```python
from build123d import *

# Parameters (mm, degrees)
F2_R        = 2.8448
F3_DEPTH    = 7.5184
F2_R_2      = 6.35
F4_DEPTH    = 7.5184
F5_R        = 5.08
F6_T1_DEPTH = 7.5184
F9_DEPTH    = 0.508


# Not quite as in the source:
# - a fillet or chamfer that OpenCascade refuses, or shapes differently, is made with other operations: its cross-section is extruded or revolved along the edge and cut away or added
# - two fillets or chamfers of one size are made in one step


with BuildPart() as f1:
    # F0 (on Front) → F1 (revolve)
    with BuildSketch(Plane.XZ):
        with BuildLine():
            Line((32.385, 31.75), (0, 31.75))
            Line((0, 31.75), (0, 28.575))
            Line((0, 28.575), (32.4854701757, 28.575))
            Line((32.4854701757, 28.575), (35.56, 25.49819462))
            Line((35.56, 25.49819462), (35.56, 8.8277412578))
            Line((35.56, 8.8277412578), (39.5224, 4.572))
            Line((39.5224, 4.572), (39.5224, 0))
            Line((39.5224, 0), (43.053, 0))
            Line((43.053, 0), (43.053, -0.508))
            Line((43.053, -0.508), (44.069, -0.508))
            Line((44.069, -0.508), (44.069, 7.5184))
            Line((44.069, 7.5184), (40.8266418362, 7.5184))
            Line((40.8266418362, 7.5184), (38.735, 9.7710676491))
            Line((38.735, 9.7710676491), (38.735, 25.4))
            ThreePointArc((38.735, 25.4), (36.8751280605, 29.8901280605), (32.385, 31.75))
        make_face()
    revolve(axis=Axis((0, 0, 30.1625), (0, 0, 1)))

    # F2 (on face) → F3 (join)
    with BuildSketch(Plane(origin=(0, 0, 0), x_dir=(1, 0, 0), z_dir=(0, 0, -1))):
        with BuildLine():
            ThreePointArc((4.7616218936, 42.7888743243), (5.939646413, 44.7443151405), (6.35, 46.99))
            ThreePointArc((6.35, 46.99), (-2.2456848595, 52.929646413), (-4.7616218936, 42.7888743243))
            ThreePointArc((-4.7616218936, 42.7888743243), (0, 43.053), (4.7616218936, 42.7888743243))
        make_face()
        with Locations((0, 46.99)):
            Circle(F2_R, mode=Mode.SUBTRACT)
    extrude(amount=-F3_DEPTH)

    # F2 (on face) → F4 (join)
    with BuildSketch(Plane(origin=(0, 0, 0), x_dir=(1, 0, 0), z_dir=(0, 0, -1))):
        with Locations((0, 46.99)):
            Circle(F2_R_2)
        with Locations((0, 46.99)):
            Circle(F2_R, mode=Mode.SUBTRACT)
        with Locations((4.699, -46.7544596696)):
            Circle(F2_R_2)
        with Locations((4.699, -46.7544596696)):
            Circle(F2_R, mode=Mode.SUBTRACT)
    extrude(amount=-F4_DEPTH)

    # F5
    f5_edges = [f1.edges().sort_by_distance(p)[0] for p in [
        (9.795498, 42.966557, 3.7592),
        (-1.049351, 44.056505, 3.7592),
    ]]
    fillet(f5_edges, radius=F5_R)

    # F6: fillet of radius 5.08 on 2 edges, made by hand

    # F6_s2 → F6_t1 (join)
    with BuildSketch(Plane.XY):
        with BuildLine():
            ThreePointArc((10.2222959919, -42.8670202563), (7.5289917798, -44.5196041815), (6.3336992457, -47.444701952))
            ThreePointArc((6.3336992457, -47.444701952), (6.1774395627, -45.5197141608), (5.4497416206, -43.7307337838))
            ThreePointArc((5.4497416206, -43.7307337838), (7.8479099763, -43.3645831296), (10.2222959919, -42.8670202563))
        make_face()
        with BuildLine():
            ThreePointArc((-10.2222959919, -42.8670202563), (-7.5289917798, -44.5196041815), (-6.3336992457, -47.444701952))
            ThreePointArc((-6.3336992457, -47.444701952), (-6.1774395627, -45.5197141608), (-5.4497416206, -43.7307337838))
            ThreePointArc((-5.4497416206, -43.7307337838), (-7.8479099763, -43.3645831296), (-10.2222959919, -42.8670202563))
        make_face()
    extrude(amount=F6_T1_DEPTH)

    # F8 (on face) → F9 (cut)
    with BuildSketch(Plane(origin=(0, 0, 0), x_dir=(1, 0, 0), z_dir=(0, 0, -1))):
        with BuildLine():
            Line((11.2232032022, 41.5248573346), (11.5476018718, 42.6009083999))
            ThreePointArc((11.5476018718, 42.6009083999), (0.1217283712, 44.1331880413), (-11.3123981282, 42.6637604833))
            Line((-11.3123981282, 42.6637604833), (-10.9422300011, 41.5995270014))
            ThreePointArc((-10.9422300011, 41.5995270014), (0.145362907, 43.0097069155), (11.2232032022, 41.5248573346))
        make_face()
        with BuildLine():
            Line((-7.2390749119, -42.3223562539), (-7.4246343474, -43.5135134363))
            ThreePointArc((-7.4246343474, -43.5135134363), (4.1004463869, -43.9625847646), (15.3315616772, -41.3374751806))
            Line((15.3315616772, -41.3374751806), (14.8499479477, -40.2801455114))
            ThreePointArc((14.8499479477, -40.2801455114), (3.9400511762, -42.757274104), (-7.2390749119, -42.3223562539))
        make_face()
    extrude(amount=F9_DEPTH, mode=Mode.SUBTRACT)


solid = f1.part
```
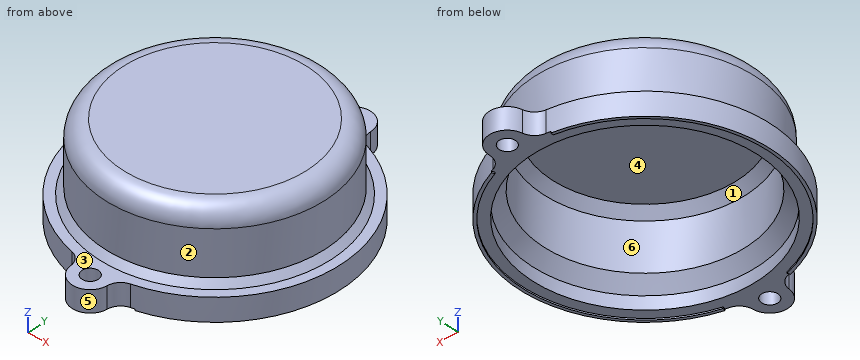
Input: part model. Units: mm. Frame: model coordinates. Face numbers are marked on the shaded views. A direction names the side the tool comes from. Coordinates: 2 decimals unless noted, no trailing zeros. Loops run counter-clockwise (first coordinate to the right, second up) from the corner with the lowest first, then second, coordinate; pieces in that order, holes last. Notation, with made-up numbers: M -5,-13.5 L 29,-13.5 A28 ccw 29,14.5 Z; hole C -35,47.25 d3. An arc over 180 degrees is marked long. Use a Markdown table: item, result. Add a question column.
1) Line query: L1, parallel to Y at x = 0, z = 19 (3 decimals); L2, parallel to Z at x = 12.5, y = -15 (3 decimals); L3, parallel to Z at x = 26.5, y = 33. Output: solid intervals per line, ascending. Write a range as from..to.
2) Set-up query: the marked faces 5 and 6. Return all of +Z, -Z, +X, -X, +Y, -Y with unobstructed straight access to the full face (end or side cutting, diameter ignored); none if empty.
3) Section B-B, the plane x = 0. Return the cut outline in (y, z) (3 decimals).
4) Section A-A, the plane y = 0. Return the cut outline in (x, z) (3 decimals), plus the area to 3 significant figures.
5) Draft query along Y for the marked faces 1, 2, 3 and 4. Return one class per face: +Y half, -Y half, draft (parallel to the pull), parting line (faces both ways), or undercut.
6) Pin query (flat end, axial travel): P1, Ø4, axis at x = -9.5, z = 23, coming from the -Y side; P2, Ø12, axis at y = -40.5, z = 26.5, coming from the -X side; P3, Ø4, axis at x = 12.5, z = 3.5, coming from the +Y side; P4, Ø3.5, axis at x = 4.7, y = 46.75, coming from the -Z side. Return the tip coordinate at first contact, or that it passes through.
7) Section C-C, the plane z = 19.5. Return the cut outline in (x, y) (3 decimals), plus the area to 3 significant figures.
Answer below:
| question | item | result |
|---|---|---|
| 1 | L1 | -38.735..-35.56, 35.56..38.735 |
| 1 | L2 | 28.575..31.75 |
| 1 | L3 | 0..7.52 |
| 2 | face 5 | +Z, -Z, -Y |
| 2 | face 6 | -Z |
| 3 | outline | M -53.34,0 L -49.835,0 L -49.835,7.518 L -53.34,7.518 Z; M -44.145,0 L -39.522,0 L -39.522,4.572 L -35.56,8.828 L -35.56,25.498 L -32.485,28.575 L 32.485,28.575 L 35.56,25.498 L 35.56,8.828 L 39.522,4.572 L 39.522,0 L 51.026,0 L 51.026,7.518 L 40.827,7.518 L 38.735,9.771 L 38.735,25.4 A6.35 ccw 32.385,31.75 L -32.385,31.75 A6.35 ccw -38.735,25.4 L -38.735,9.771 L -40.827,7.518 L -44.145,7.518 Z |
| 4 | outline | M -44.069,-0.508 L -43.053,-0.508 L -43.053,0 L -39.522,0 L -39.522,4.572 L -35.56,8.828 L -35.56,25.498 L -32.485,28.575 L 32.485,28.575 L 35.56,25.498 L 35.56,8.828 L 39.522,4.572 L 39.522,0 L 43.053,0 L 43.053,-0.508 L 44.069,-0.508 L 44.069,7.518 L 40.827,7.518 L 38.735,9.771 L 38.735,25.4 A6.35 ccw 32.385,31.75 L -32.385,31.75 A6.35 ccw -38.735,25.4 L -38.735,9.771 L -40.827,7.518 L -44.069,7.518 Z |
| 4 | area | 452 mm2 |
| 5 | face 1 | undercut |
| 5 | face 2 | parting line |
| 5 | face 3 | draft |
| 5 | face 4 | undercut |
| 6 | P1 | y = -38 |
| 6 | P2 | x = -17.51 |
| 6 | P3 | y = 49.34 |
| 6 | P4 | through |
| 7 | outline | C 0,0 d77.47; hole C 0,0 d71.12 |
| 7 | area | 741 mm2 |
